The listing builds one solid part. Answer for the finished solid, in the listing's coordinates (mm). A direction names the side the tool comes from. Round coordinates to 2 decimals unless told otherwise and drop trailing zeros. Loops run counter-clockwise (first coordinate to the right, second up) from the corner with the lowest first, then second, coordinate; pieces in that order, holes last. Notation, with made-up numbers: M 33,27 L 87,27 A19 ccw 87,39 Z; hole C 55,42 d10. An arc over 180 degrees is marked long. Answer as a JSON object with one key per item and string values.
Autodesk Inventor part; units mm, degrees
ref_plane "Work Plane1" through (0, 0, -15) normal (0, 0, 1) x (1, 0, 0)
ref_plane "YZ Plane" through (0, 0, 0) normal (1, 0, 0) x (0, 1, 0)
ref_plane "XZ Plane" through (0, 0, 0) normal (0, 1, 0) x (-1, 0, 0)
sketch "Sketch1" plane through (0, 0, 0) normal (0, 0, 1) x (1, 0, 0)
  line L0 (0, 0) -> (25, 0)
  line L1 (25, 0) -> (25, 40)
  line L2 (25, 40) -> (0, 40)
  line L3 (0, 40) -> (0, 0)
  dimension "d1" = 25
  dimension "d2" = 40
  dimension "d3" = 25
extrude "Extrusion1" add sketch "Sketch1" against normal blind 30
sketch "Sketch2" plane through (25, 0, 0) normal (1, 0, 0) x (0, 0, -1)
  line L0 (0, 0) -> (30, 0)
  circle A0 centre (15, 6.56) radius 2.46
extrude "Extrusion2" cut sketch "Sketch2" against normal blind 30
sketch "Sketch3" plane through (0, 0, 0) normal (-1, 0, 0) x (0, 0, 1)
  line L0 (0, 0) -> (-30, 0)
  line L1 (-25.05, 0) -> (-4.95, 0)
  line L2 (-4.95, 0) -> (-4.95, 33.12)
  line L3 (-4.95, 33.12) -> (-25.05, 33.12)
  line L4 (-25.05, 33.12) -> (-25.05, 0)
  dimension "d11" = 20.1
extrude "Extrusion3" cut sketch "Sketch3" against normal blind 20
sketch "Sketch4" plane through (0, 0, 0) normal (0, -1, 0) x (1, 0, 0)
  line L0 (20, -4.95) -> (20, -25.05)
  line L1 (20, -15) -> (25, -15)
  line L2 (25, 0) -> (25, -30)
  line L3 (20, -8.025) -> (25, -8.025)
  line L4 (25, -8.025) -> (25, -21.975)
  line L5 (25, -21.975) -> (20, -21.975)
  line L6 (20, -21.975) -> (20, -8.025)
  line L7 (20, -8.025) -> (25, -21.975) construction
  line L8 (25, -8.025) -> (20, -21.975) construction
  line L9 (25, -12.54) -> (25, -17.46)
  point P0 (0, 0)
  point P1 (22.5, -15)
  dimension "d14" = 13.95
extrude "Extrusion4" add sketch "Sketch4" along normal blind 15
sketch "Sketch5" plane through (20, 0, 0) normal (-1, 0, 0) x (0, 0, 1)
  circle A0 centre (-15, 6.56) radius 2.46
  circle A1 centre (-15, 6.56) radius 4.7025
  circle A2 centre (-15, 6.56) radius 2.46
  circle A3 centre (-15, 6.56) radius 2.46
  point P0 (0, 0)
  dimension "d17" = 9.405
extrude "Extrusion5" cut sketch "Sketch5" against normal blind 2.1
sketch "Sketch6" plane through (25, 0, 0) normal (1, 0, 0) x (0, 0, -1)
  circle A0 centre (15, 6.56) radius 4.7025
  line L0 (15, 6.56) -> (15, 23.56)
  circle A1 centre (15, 23.56) radius 2.46
  point P0 (0, 0)
  dimension "d20" = 17
  dimension "d21" = 4.92
extrude "Extrusion6" cut sketch "Sketch6" against normal blind 10 contours A1
sketch "Sketch7" plane through (20, 0, 0) normal (-1, 0, 0) x (0, 0, 1)
  circle A0 centre (-15, 23.56) radius 2.46
  circle A1 centre (-15, 23.56) radius 4.7025
  point P0 (0, 0)
  dimension "d24" = 9.405
extrude "Extrusion7" cut sketch "Sketch7" against normal blind 2.1
sketch "Sketch9" plane through (25, 0, 0) normal (1, 0, 0) x (0, 0, -1)
  circle A0 centre (15, 6.56) radius 2.46
  circle A1 centre (15, 6.56) radius 2.46
  circle A2 centre (15, 23.56) radius 2.46
  circle A3 centre (15, 23.56) radius 2.46
  line L0 (30, 40) -> (30, 0)
  line L1 (30, 0) -> (30, 40)
  line L2 (30, 40) -> (0, 40)
  line L3 (0, 40) -> (0, 0)
  line L4 (0, 0) -> (8.025, 0)
  line L5 (21.975, 0) -> (21.975, -15)
  line L6 (21.975, -15) -> (8.025, -15)
  line L7 (8.025, -15) -> (8.025, 0)
  line L8 (0, 0) -> (8.025, 0)
  line L9 (21.975, 0) -> (30, 0)
extrude "Extrusion8" add sketch "Sketch9" along normal blind 5
sketch "Sketch10" plane through (0, 40, 0) normal (0, 1, 0) x (1, 0, 0)
  line L0 (0, 30) -> (30, 30)
  line L1 (30, 0) -> (0, 0)
  line L2 (0, 30) -> (30, 30)
  line L3 (30, 30) -> (30, 0)
  line L4 (30, 0) -> (0, 0)
  line L5 (0, 0) -> (0, 30)
extrude "Extrusion9" add sketch "Sketch10" along normal blind 30
sketch "Sketch12" plane through (30, 0, 0) normal (1, 0, 0) x (0, 0, -1)
  circle A0 centre (15, 6.56) radius 2.46
  line L0 (15, 6.56) -> (15, 15.06)
  circle A1 centre (15, 15.06) radius 2.525
  point P0 (0, 0)
  dimension "d31" = 8.5
  dimension "d33" = 5.05
extrude "Extrusion10" cut sketch "Sketch12" against normal blind 30 contours A1
sketch "Sketch14" plane through (0, 0, 0) normal (0, 0, 1) x (1, 0, 0)
  line L0 (30, 70) -> (0, 70)
  line L1 (0, 70) -> (0, 85)
  line L2 (-15, 100) -> (-23, 100)
  line L3 (30, 0) -> (30, 70)
  line L4 (30, 109) -> (30, 70)
  arc A0 (0, 85) -> (-15, 100) centre (-15, 85) ccw
  line L5 (30, 105) -> (30, 100)
  line L6 (-23, 124) -> (15, 124)
  line L7 (-19, 122) -> (-23, 124)
  line L8 (-19, 122) -> (-15, 112)
  line L9 (-19, 102) -> (-23, 100)
  line L10 (-19, 102) -> (-15, 112)
  line L11 (30, 109) -> (15, 124)
  point P0 (0, 0)
  point P1 (0, 100)
  dimension "d47" = 30
  dimension "d54" = 15
extrude "Extrusion12" add sketch "Sketch14" against normal blind 30
sketch "Sketch15" plane through (0, 0, -25.05) normal (-1, 0, 0) x (0, 0, 1)
  line L0 (0, 33.12) -> (20.1, 33.12)
  line L1 (20.1, 33.12) -> (20.1, 0)
  line L2 (0, 33.12) -> (20.1, 33.12)
  line L3 (20.1, 33.12) -> (20.1, 31.1)
  line L4 (20.1, 31.1) -> (0, 31.1)
  line L5 (0, 31.1) -> (0, 33.12)
  point P0 (25.05, 0)
  dimension "d57" = 2.02
extrude "Extrusion13" add sketch "Sketch15" against normal blind 20
sketch "Sketch19" plane through (0, 0, 0) normal (0, 0, 1) x (1, 0, 0)
  arc A0 (0, 85) -> (-15, 100) centre (-15, 85) ccw
  arc A1 (0, 85) -> (-15, 100) centre (-15, 85) ccw
  line L0 (-15, 100) -> (-23, 100)
  line L1 (-15, 100) -> (-23, 100)
  line L2 (-23, 100) -> (-19, 102)
  line L3 (-23, 100) -> (-19, 102)
  line L4 (-19, 102) -> (-15, 112)
  line L5 (-19, 102) -> (-15, 112)
  line L6 (-15, 112) -> (-19, 122)
  line L7 (-15, 112) -> (-19, 122)
  line L8 (-19, 122) -> (-23, 124)
  line L9 (-19, 122) -> (-23, 124)
  line L10 (-23, 124) -> (15, 124)
  line L11 (-23, 124) -> (15, 124)
  line L12 (15, 124) -> (30, 109)
  line L13 (15, 124) -> (30, 109)
  line L14 (30, 109) -> (30, 85)
  line L15 (30, 0) -> (30, 109)
  line L16 (0, 85) -> (30, 85)
  point P0 (0, 0)
extrude "Extrusion14" add sketch "Sketch19" along normal blind 30
ref_plane "Work Plane1" through (0, 0, -15) normal (0, 0, 1) x (1, 0, 0)
mirror "Mirror1" about plane through (0, 0, -15) normal (0, 0, 1) of "Extrusion14"
properties part number "20mm_x_90mm"
Item 1: Which of the six approach directions +Z, -Z, +X, -X, +Y, -Y give full straight-line access (tool end or side, diameter ignored) to faces 4 (the face through (25, -8, -8.025)), 5 (the face through (22.1, 4.5, -13)), 6 (the face through (15, 43, -30)), 7 (the face through (-17, 117, -14)), 8 (the face through (20, 8, -20))?
Values follow:
{"face 4": "+Z, +X, -X, -Y", "face 5": "-X", "face 6": "-Z, +X, -X, -Y", "face 7": "+Z, -Z, -X", "face 8": "-X, -Y"}
Item 2: The part is cut by section A-A (y = 23.56). Give the vertices of the cut face in (x, z).
Values follow:
{"outline": "M 0,-30 L 30,-30 L 30,-17.46 L 22.1,-17.46 L 22.1,-19.7 L 20,-19.7 L 20,-25.05 L 0,-25.05 Z; M 0,-4.95 L 20,-4.95 L 20,-10.3 L 22.1,-10.3 L 22.1,-12.54 L 30,-12.54 L 30,0 L 0,0 Z"}
Item 3: The part is cut by section D-D (x = 18.5). Give the vertices of the cut face in (y, z), then the cut area to 3 significant figures.
Values follow:
{"outline": "M 0,-30 L 85,-30 L 85,-60 L 120.5,-60 L 120.5,30 L 85,30 L 85,0 L 0,0 L 0,-4.95 L 31.1,-4.95 L 31.1,-25.05 L 0,-25.05 Z", "area": "5,120 mm^2"}
Item 4: Determine the mould class of faces 1 (the face through (22.1, 21.5, -13)), 2 (the face through (10, 16, -25.05)), 3 (the face through (25, -15, -15)) for opening direction Y: released by +Y, released by -Y, zero draft, split by the parting line, or undercut.
Values follow:
{"face 1": "undercut", "face 2": "zero draft", "face 3": "released by -Y"}
Item 5: The part is cut by section C-C (z = -15). Give the number of separate pieces and of enclosed holes in the cut face, then the cut area to 3 significant figures.
Values follow:
{"separate pieces": "4", "enclosed holes": "0", "area": "3,440 mm^2"}
Item 6: Straight lines are drawn through the part: line 1 (Z direction, x = 23.5, y = 15.06) (3 decimals); line 2 (Y direction, x = 26, z = -15) (3 decimals); line 3 (Y direction, x = 24, z = -15) (3 decimals). For each, find the intervals that lie inside material, in ascending order.
Values follow:
{"line 1": "-30 to -17.525, -12.475 to 0", "line 2": "-15 to 4.1, 9.02 to 12.535, 17.585 to 21.1, 26.02 to 113", "line 3": "-15 to 4.1, 9.02 to 12.535, 17.585 to 21.1, 26.02 to 115"}
Item 7: The part is cut by section B-B (x = 25.5). Give the vertices of the cut face in (y, z) (3 decimals), then the cut area to 3 significant figures.
Values follow:
{"outline": "M -15,-21.975 L 0,-21.975 L 0,-30 L 85,-30 L 85,-60 L 113.5,-60 L 113.5,30 L 85,30 L 85,0 L 0,0 L 0,-8.025 L -15,-8.025 Z; hole C 6.56,-15 d4.92; hole C 15.06,-15 d5.05; hole C 23.56,-15 d4.92", "area": "5,270 mm^2"}
Item 8: Flat-ended cylindrical pins translate along their axes: P1, Ø16, axis at x = 15, y = 15, coming from the -Z side; P2, Ø10, axis at y = 0.5, z = -14.5, coming from the -X side; P3, Ø4, axis at y = 108, z = -6.5, coming from the -X side; P4, Ø4.5, axis at y = 6.56, z = -15, coming from the -X side. Find the tip coordinate at first contact, or state that the pin passes through.
Values follow:
{"P1": "z = -30", "P2": "x = 20", "P3": "x = -17.4", "P4": "through"}
